```python
from build123d import *

# Parameters (mm, degrees)
CROQUIS1_W              = 23
CROQUIS1_H              = 12
SALIENTE_EXTRUIR1_DEPTH = 23.2
CROQUIS6_R              = 2
CORTAR_EXTRUIR1_DEPTH   = 0.5
SALIENTE_EXTRUIR3_DEPTH = 4.1
CROQUIS8_R              = 2.5
SALIENTE_EXTRUIR4_DEPTH = 4
CROQUIS9_R              = 0.5
CORTAR_EXTRUIR2_DEPTH   = 4
CROQUIS11_W             = 12
CROQUIS11_H             = 3
SALIENTE_EXTRUIR5_DEPTH = 4.75
CORTAR_EXTRUIR3_DEPTH   = 3
CHAFL_N3_SIZE           = 1


with BuildPart() as part:
    # Croquis1 → Saliente-Extruir1 (new body)
    with BuildSketch(Plane(origin=(0, 0, 0), x_dir=(1, 0, 0), z_dir=(0, 1, 0))):
        Rectangle(CROQUIS1_W, CROQUIS1_H)
    saliente_extruir1 = extrude(amount=SALIENTE_EXTRUIR1_DEPTH)

    # Croquis6 → Cortar-Extruir1 (cut)
    with BuildSketch(Plane.XZ):
        with Locations((-11.5, 6)):
            Circle(CROQUIS6_R)
        with Locations((11.5, 6)):
            Circle(CROQUIS6_R)
        with Locations((-11.5, -6)):
            Circle(CROQUIS6_R)
        with Locations((11.5, -6)):
            Circle(CROQUIS6_R)
    extrude(amount=-CORTAR_EXTRUIR1_DEPTH, mode=Mode.SUBTRACT)

    # Croquis7 → Saliente-Extruir3 (add)
    with BuildSketch(Plane(origin=(0, 23.2, 0), x_dir=(1, 0, 0), z_dir=(0, 1, 0))):
        with BuildLine():
            ThreePointArc((0.020833333, -2.445144707), (11.5, 0), (0.020833333, 2.445144707))
            ThreePointArc((0.020833333, 2.445144707), (-3, 0), (0.020833333, -2.445144707))
        make_face()
    extrude(amount=SALIENTE_EXTRUIR3_DEPTH)

    # Croquis8 → Saliente-Extruir4 (add)
    with BuildSketch(Plane(origin=(0, 27.3, 0), x_dir=(1, 0, 0), z_dir=(0, 1, 0))):
        with Locations(Location((5.5, 0, 0), (0, 0, 270))):
            Circle(CROQUIS8_R)
    extrude(amount=SALIENTE_EXTRUIR4_DEPTH)

    # Croquis9 → Cortar-Extruir2 (cut)
    with BuildSketch(Plane(origin=(0, 31.3, 0), x_dir=(1, 0, 0), z_dir=(0, 1, 0))):
        with Locations(Location((5.5, 0, 0), (0, 0, 270))):
            Circle(CROQUIS9_R)
    extrude(amount=-CORTAR_EXTRUIR2_DEPTH, mode=Mode.SUBTRACT)

    # Croquis11 → Saliente-Extruir5 (add)
    with BuildSketch(Plane.ZY.offset(11.5)):
        with Locations((0, 17.89988551)):
            Rectangle(CROQUIS11_W, CROQUIS11_H)
    saliente_extruir5 = extrude(amount=SALIENTE_EXTRUIR5_DEPTH)

    # Croquis12 → Cortar-Extruir3 (cut)
    with BuildSketch(Plane(origin=(0, 19.39988551, 0), x_dir=(1, 0, 0), z_dir=(0, 1, 0))):
        with BuildLine():
            Line((-16.25, 0.5), (-15.079795897, 0.5))
            ThreePointArc((-15.079795897, 0.5), (-13, 0), (-15.079795897, -0.5))
            Line((-15.079795897, -0.5), (-16.25, -0.5))
            Line((-16.25, -0.5), (-16.25, 0.5))
        make_face()
    cortar_extruir3 = extrude(amount=-CORTAR_EXTRUIR3_DEPTH, mode=Mode.SUBTRACT)

    # Simetría1: Saliente-Extruir1, Saliente-Extruir5, Cortar-Extruir3 across plane
    add(saliente_extruir1.mirror(Plane.ZY))
    add(saliente_extruir5.mirror(Plane.ZY))
    add(cortar_extruir3.mirror(Plane.ZY), mode=Mode.SUBTRACT)

    # Chaflán3
    chafl_n3_edges = [part.edges().sort_by_distance(p)[0] for p in [
        (11.5, 8.199942755, -6),
        (11.5, 8.199942755, 6),
        (-11.5, 8.199942755, 6),
        (-11.5, 8.199942755, -6),
        (-11.5, 21.299942755, -6),
        (11.5, 21.299942755, -6),
        (11.5, 21.299942755, 6),
        (-11.5, 21.299942755, 6),
    ]]
    chamfer(chafl_n3_edges, length=CHAFL_N3_SIZE)


solid = part.part
```
CAD build for the part. Positions are in the model's coordinates, mm. A direction names the side the tool comes from. Give positions to 0.01 mm unless a question says otherwise; leave off trailing zeros. Write each loop counter-clockwise with the first axis right and the second up, starting at its lowest first coordinate (ties: lowest second). Pieces come first, ordered by that corner, then holes. Notation, with made-up numbers: M 45,26.25 L 49,26.25 A22 cw 49,43.25 Z; hole C 79.25,43 d5. An arc over 180 degrees is marked long. Return JSON: item names as keys, results as strings. Group by question number.
(1) Band-saw the part on A-A (x = 14.1). Give the cut face in (y, z), and give its area (3 significant figures).
(2) Drill centre lines: L1, parallel to Z at x = 14.1, y = 18.35; L2, parallel to X at y = 29.65, z = 0; L3, parallel to Y at x = 0, z = -3. Where is each one in solid material? Low to high. Write a range as [from, to].
(3) Band-saw the part on D-D (y = 29.5). Give the cut face in (x, z), and give its area (3 significant figures).
(4) Band-saw the part on C-C (x = -0.5). Give the cut face in (y, z).
(5) Flat gauge pins, fed straight in: pin 1 Ø5 at (y, z) = (26, 1.5) entering from +X; pin 2 Ø1.7 at (x, z) = (13.5, -2.5) entering from +Y; pin 3 Ø2 at (x, z) = (14.1, 0) entering from +Y; pin 4 Ø2 at (y, z) = (24, 3) entering from -X. Where does each tip first touch, or does it go through?
(6) 3-axis set-ups, long thin cutter, end or side, ignore diameter. For faces 1 (the face through (16, 18, -0.5)), 2 (the face through (-11, 21.3, 5.5)), 3 (the face through (5, 29, 0)), 4 (the face through (11, 21.3, 5.5)), 5 (the face through (-16, 18, -0.5)): which of +Z, -Z, +X, -X, +Y, -Y reach the whole face in a straight line?
(7) Band-saw the part on B-B (y = 8.5). Give the cut face in (x, z), and give its area (3 significant figures).
Entries:
{
 "1": {"outline": "M 16.4,-6 L 19.4,-6 L 19.4,-1.1 L 16.4,-1.1 Z; M 16.4,1.1 L 19.4,1.1 L 19.4,6 L 16.4,6 Z", "area": "29.4 mm^2"},
 "2": {"L1": "z = [-6, -1.1], [1.1, 6]", "L2": "x = [3, 5], [6, 8]", "L3": "y = [0, 23.2]"},
 "3": {"outline": "C 5.5,0 d5; hole C 5.5,0 d1", "area": "18.8 mm^2"},
 "4": {"outline": "M 0,-6 L 23.2,-6 L 23.2,-2.5 L 27.3,-2.5 L 27.3,2.5 L 23.2,2.5 L 23.2,6 L 0,6 Z"},
 "5": {"pin 1": "stops at x = 11.5", "pin 2": "stops at y = 19.4", "pin 3": "passes through", "pin 4": "stops at x = -11.5"},
 "6": {"face 1": "+X, +Y, -Y", "face 2": "+Z, -X, +Y", "face 3": "+Y", "face 4": "+Z, +X, +Y", "face 5": "-X, +Y, -Y"},
 "7": {"outline": "M -11.5,-5 L -10.5,-6 L 10.5,-6 L 11.5,-5 L 11.5,5 L 10.5,6 L -10.5,6 L -11.5,5 Z", "area": "274 mm^2"}
}
